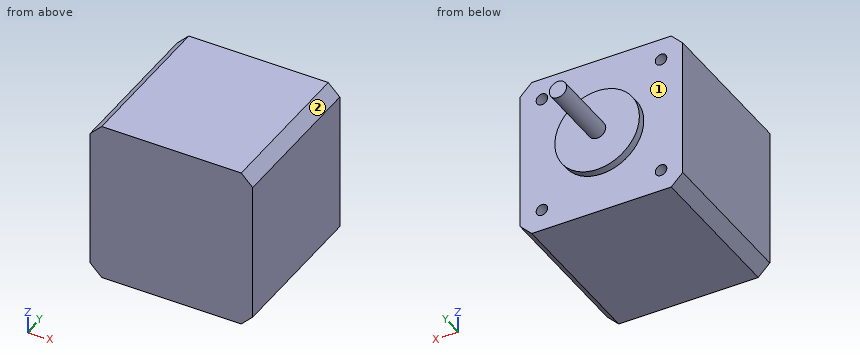
Autodesk Fusion 360 part; units mm, degrees
sketch "スケッチ1" plane through (0, 0, 0) normal (0, 1, 0) x (1, 0, 0)
  line L0 (0, 0) -> (21.15, 0)
  line L1 (21.15, 0) -> (21.15, 21.15)
  line L2 (21.15, 21.15) -> (0, 21.15)
  line L3 (0, 21.15) -> (0, 0)
  line L4 (0, 0) -> (15.5, 0) construction
  line L5 (15.5, 0) -> (15.5, 15.5) construction
  line L6 (15.5, 15.5) -> (0, 15.5) construction
  line L7 (0, 15.5) -> (0, 0) construction
  circle A0 centre (15.5, 15.5) radius 1.5
  dimension "d1" = 21.15
  dimension "d2" = 21.15
  dimension "d3" = 15.5
  dimension "d4" = 15.5
  dimension "d5" = 3
extrude "押し出し1" add sketch "スケッチ1" along normal blind 40 contours L0 L1 L2 L3 | A0 makes body 1
mirror "ミラー1" about plane through (0, 0, 0) normal (0, 0, 1) of bodies 1 makes body 2
mirror "ミラー2" about plane through (0, 0, 21.15) normal (-1, 0, 0) of bodies 1 2 makes body 3 at (0, 13.3333, -14.1) makes body 4 at (0, 13.3333, 14.1)
combine "結合1" operation add target body 4 tool bodies 1 2 3
sketch "スケッチ2" plane through (0, 40, 0) normal (0, 1, 0) x (-1, 0, 0)
  line L0 (-21.15, -21.15) -> (21.15, -21.15)
  line L1 (21.15, -21.15) -> (21.15, 21.15)
  line L2 (21.15, 21.15) -> (-21.15, 21.15)
  line L3 (-21.15, 21.15) -> (-21.15, -21.15)
  circle A0 centre (0, 0) radius 11
  line L4 (15.5, 15.5) -> (-15.5, 15.5) construction
  line L5 (-15.5, 15.5) -> (-15.5, -15.5) construction
  line L6 (-15.5, -15.5) -> (15.5, -15.5) construction
  line L7 (15.5, -15.5) -> (15.5, 15.5) construction
  line L8 (15.5, 15.5) -> (-15.5, -15.5) construction
  line L9 (-15.5, 15.5) -> (15.5, -15.5) construction
  circle A1 centre (15.5, -15.5) radius 1.5
  circle A2 centre (-15.5, -15.5) radius 1.5
  circle A3 centre (15.5, 15.5) radius 1.5
  circle A4 centre (-15.5, 15.5) radius 1.5
  circle A5 centre (0, 0) radius 2.25
  dimension "d10" = 22
  dimension "d13" = 31
  dimension "d14" = 31
  dimension "d15" = 3
  dimension "d16" = 3
  dimension "d17" = 3
  dimension "d18" = 3
  dimension "d21" = 4.5
extrude "押し出し2" add sketch "スケッチ2" along normal blind 2 contours A0 | A5 bodies 4
extrude "押し出し3" cut sketch "スケッチ2" against normal blind 4.5 contours A1 | A2 | A3 | A4 bodies 4
extrude "押し出し4" add sketch "スケッチ2" along normal blind 20 contours A5 bodies 4
chamfer "面取り1" distance 3 angle 45 4 edges at (-21.15, 20, -21.15) (-21.15, 20, 21.15) (21.15, 20, 21.15) (21.15, 20, -21.15) on bodies 4
equation "d1 = ( 42.3 / 2 ) * 1 mm"
equation "d2 = ( 42.3 / 2 ) * 1 mm"
equation "d3 = ( 31 / 2 ) * 1 mm"
equation "d4 = ( 31 / 2 ) * 1 mm"
Input: part model. Units: mm. Frame: model coordinates. Face numbers are marked on the shaded views. A direction names the side the tool comes from. Round coordinates to 2 decimals unless told otherwise and drop trailing zeros. Loops run counter-clockwise (first coordinate to the right, second up) from the corner with the lowest first, then second, coordinate; pieces in that order, holes last. Notation, with made-up numbers: (7, 12) -> (36, 12) arc R29 ccw to (36, 40) -> close; hole circle Ø9 at (78.25, 24.5). An arc over 180 degrees is marked (long way). One line per item, written item: value.
(1) Section D-D (z = 12.5). Return the cut outline in (x, y), plus the area to 3 significant figures.
Geometry check:
outline: (-21.15, 0) -> (21.15, 0) -> (21.15, 40) -> (-21.15, 40) -> close
area: 1,690 mm2
(2) Section B-B (z = -15.5). Return the cut outline in (x, y).
Geometry check:
outline: (-21.15, 0) -> (21.15, 0) -> (21.15, 40) -> (17, 40) -> (17, 35.5) -> (14, 35.5) -> (14, 40) -> (-14, 40) -> (-14, 35.5) -> (-17, 35.5) -> (-17, 40) -> (-21.15, 40) -> close
(3) Section A-A (x = 0). Return the cut outline in (y, z), plus the area to 3 significant figures.
Geometry check:
outline: (0, -21.15) -> (40, -21.15) -> (40, -11) -> (42, -11) -> (42, -2.25) -> (60, -2.25) -> (60, 2.25) -> (42, 2.25) -> (42, 11) -> (40, 11) -> (40, 21.15) -> (0, 21.15) -> close
area: 1,820 mm2
(4) Material intervals for line 1 (Z direction, x = 15.5, y = 36.6); line 2 (X direction, y = 38, z = -15), sorted ascending. Write a range as [from, to].
Geometry check:
line 1: [-21.15, -17], [-14, 14], [17, 21.15]
line 2: [-21.15, -16.91], [-14.09, 14.09], [16.91, 21.15]
(5) Set-up query: the marked faces 1 and 2. Return all of +Z, -Z, +X, -X, +Y, -Y with unobstructed straight access to the full face (end or side cutting, diameter ignored); none if empty.
Geometry check:
face 1: +Y
face 2: +Z, +X, +Y, -Y
(6) Pin query (flat end, axial travel): pin 1 (1.5 mm diameter, centred on x = -15.5, z = -15, fed in from +Y); pin 2 (2.5 mm diameter, centred on x = -16, z = 15, fed in from +Y); pin 3 (1.5 mm diameter, centred on x = 2.5, y = 42.5, fed in from +Z). Return the tip coordinate at first contact, or that it passes through.
Geometry check:
pin 1: y = 35.5
pin 2: y = 40
pin 3: z = 10.83
(7) Section C-C (y = 48). Return the cut outline in (x, z), plus the area to 3 significant figures.
Geometry check:
outline: circle Ø4.5 at (0, 0)
area: 15.9 mm2
